```python
from build123d import *

# Parameters (mm, degrees)
EXTRUDE_1_DEPTH = 4


with BuildPart() as part:
    # Эскиз1 → Бобышка-Вытянуть1 (new body)
    with BuildSketch(Plane.XY):
        with BuildLine():
            Line((-82.424778316, -3.697860687), (-73.838144401, -3.697860687))
            Line((-73.838144401, -3.697860687), (-73.838144401, -46.859686904))
            add(Edge.make_bspline(
                [(-83.795378854, -32.554799456), (-82.720974338, -42.41019878), (-73.838144401, -46.859686904)],
                knots=[0, 0, 0, 1, 1, 1], degree=2))
            Line((-83.795378854, -32.554799456), (-86.424778316, -20.197860687))
            Line((-86.424778316, -20.197860687), (-82.424778316, -20.197860687))
            Line((-82.424778316, -20.197860687), (-82.424778316, -3.697860687))
        make_face()
    extrude(amount=EXTRUDE_1_DEPTH)


solid = part.part
```
The model under review builds one solid part; all positions refer to its coordinate system, in mm. A direction names the side the tool comes from. Give positions to 0.01 mm unless a question says otherwise; leave off trailing zeros. Write each loop counter-clockwise with the first axis right and the second up, starting at its lowest first coordinate (ties: lowest second). Pieces come first, ordered by that corner, then holes. Notation, with made-up numbers: (-17, -37) -> (7, -37) arc R19 cw to (7, -9) -> close; hole circle Ø7 at (77.25, -14). An arc over 180 degrees is marked (long way). Put each result on its own line as item: value.
(1) For pin 1 Ø6 at (x, y) = (-77, -9) entering from -Z; pin 2 Ø1.2 at (y, z) = (-14, 2.5) entering from -X; pin 3 Ø2 at (x, z) = (-83.5, 2.5) entering from +Y, all flat-tipped, find the tip position at first contact; note any pin that passes through.
Results are:
pin 1: z = 0
pin 2: x = -82.42
pin 3: y = -20.2
(2) We need section B-B, the plane x = -85.5. Give the boundary of the cut face in (y, z), and give its area (3 significant figures).
Results are:
outline: (-24.54, 0) -> (-20.2, 0) -> (-20.2, 4) -> (-24.54, 4) -> close
area: 17.4 mm²
(3) To check wall thickness, follow probe 1 along X at (y, z) = (-12, 1.8); probe 2 along Y at (x, z) = (-79, 0.2); probe 3 along X at (y, z) = (-36, 1.7). State the ranges of each line that lie inside material, in increasing order. Write a range as from..to.
Results are:
probe 1: -82.42..-73.84
probe 2: -43.18..-3.7
probe 3: -83.14..-73.84
(4) We need section A-A, the plane y = -19. Give the boundary of the cut face in (x, z).
Results are:
outline: (-82.42, 0) -> (-73.84, 0) -> (-73.84, 4) -> (-82.42, 4) -> close
(5) Tool access review of faces 1 (the flat face through (-84, -20.198, 2)), 2 (the flat face through (-79, -25, 4)): name each direction out of +Z, -Z, +X, -X, +Y, -Y from which nothing blocks a thin tool from reaching the whole face with its end or side.
Results are:
face 1: +Z, -Z, -X, +Y
face 2: +Z, +X, -X, +Y, -Y
